Could you check a few things on this model? Use its own coordinates, in mm. A direction names the side the tool comes from. Give positions to 0.01 mm unless a question says otherwise; leave off trailing zeros. Loops run counter-clockwise (first coordinate to the right, second up) from the corner with the lowest first, then second, coordinate; pieces in that order, holes last.
1. For faces 4 (the flat face through (0, 0, 0)), 5 (the flat face through (1.926, -2.888, 4.056)), which set-ups out of +Z, -Z, +X, -X, +Y, -Y let a thin tool reach every point of the face, with its end or its side?
2. Imagine slicing it at B-B (x = -1.75). List the corners of the cut face in (y, z) for me, plus the area to 3 significant figures.
3. Thinking about a two-plate mould opening in Y: for faces 1 (the flat face through (-3.055, -1.764, 4.056)), 2 (the flat face through (0, 0, 8)), 3 (the cylindrical face through (-1.46, -6.59, 3.94)), which applies, +Y half, -Y half, draft (parallel to the pull), parting line (faces both ways), or undercut?
4. Imagine slicing it at D-D (x = -0.25). List the corners of the cut face in (y, z) for me, plus the area to 3 significant figures.
5. For P1, Ø4, axis at x = 2.5, y = 2, coming from the -Z side; P2, Ø2, axis at x = 2.5, z = 6, coming from the -Y side; P3, Ø1, axis at y = 5, z = 3.5, coming from the -X side; P4, Ø4, axis at y = 2.5, z = 5, coming from the -X side, each with a flat end and sliding along its axis, tell me the tip position at first contact or that it passes through.
6. Imagine slicing it at A-A (z = 3.5). List the corners of the cut face in (x, y) for me.
7. I need wall thicknesses on line 1 along Y through (x, z) = (3, 4.5); line 2 along Y through (x, z) = (-4.5, 4.75); line 3 along X through (y, z) = (-3.25, 1.25). Which ranges of each line are inside material? Lowest first, please.
8. Imagine slicing it at C-C (y = -4). List the corners of the cut face in (x, z) for me.
```python
from build123d import *

# Parameters (mm, degrees)
F0_R     = 6.75
F1_DEPTH = 8
F3_DEPTH = 25


with BuildPart() as f1:
    # F0 (on Top) → F1 (new body)
    with BuildSketch(Plane.XY):
        Circle(F0_R)
    extrude(amount=F1_DEPTH)

    # F2 (on face) → F3 (cut)
    with BuildSketch(Plane.XY.offset(8)):
        with BuildLine():
            ThreePointArc((0, 1.5), (0.363208, 1.455362), (0.704799, 1.324107))
            Line((0.704799, 1.324107), (2.395915, 4.950716))
            ThreePointArc((2.395915, 4.950716), (1.229036, 5.360921), (0, 5.5))
            Line((0, 5.5), (0, 1.5))
        make_face()
        with BuildLine():
            ThreePointArc((1.299038, 0.75), (1.441985, 0.413134), (1.499109, 0.051679))
            Line((1.499109, 0.051679), (5.485404, 0.400435))
            ThreePointArc((5.485404, 0.400435), (5.257212, 1.616084), (4.76314, 2.75))
            Line((4.76314, 2.75), (1.299038, 0.75))
        make_face()
        with BuildLine():
            Line((4.76314, -2.75), (1.299038, -0.75))
            ThreePointArc((1.299038, -0.75), (1.078777, -1.042229), (0.79431, -1.272427))
            Line((0.79431, -1.272427), (3.089488, -4.550281))
            ThreePointArc((3.089488, -4.550281), (4.028175, -3.744837), (4.76314, -2.75))
        make_face()
        with BuildLine():
            Line((0, -5.5), (0, -1.5))
            ThreePointArc((0, -1.5), (-0.363208, -1.455362), (-0.704799, -1.324107))
            Line((-0.704799, -1.324107), (-2.395915, -4.950716))
            ThreePointArc((-2.395915, -4.950716), (-1.229036, -5.360921), (0, -5.5))
        make_face()
        with BuildLine():
            Line((-4.76314, -2.75), (-1.299038, -0.75))
            ThreePointArc((-1.299038, -0.75), (-1.441985, -0.413134), (-1.499109, -0.051679))
            Line((-1.499109, -0.051679), (-5.485404, -0.400435))
            ThreePointArc((-5.485404, -0.400435), (-5.257212, -1.616084), (-4.76314, -2.75))
        make_face()
        with BuildLine():
            ThreePointArc((-1.299038, 0.75), (-1.078777, 1.042229), (-0.79431, 1.272427))
            Line((-0.79431, 1.272427), (-3.089488, 4.550281))
            ThreePointArc((-3.089488, 4.550281), (-4.028175, 3.744837), (-4.76314, 2.75))
            Line((-4.76314, 2.75), (-1.299038, 0.75))
        make_face()
    extrude(amount=-F3_DEPTH, mode=Mode.SUBTRACT)


solid = f1.part
```
Derived:
1. face 4: -Z, +X, -X, +Y, -Y
1. face 5: +Z, -Z
2. outline: (-6.52, 0) - (-5.21, 0) - (-5.21, 8) - (-6.52, 8) - close; (-3.57, 0) - (-1.01, 0) - (-1.01, 8) - (-3.57, 8) - close; (-0.07, 0) - (1.01, 0) - (1.01, 8) - (-0.07, 8) - close; (2.64, 0) - (6.52, 0) - (6.52, 8) - (2.64, 8) - close
2. area: 70.6 mm2
3. face 1: undercut
3. face 2: draft
3. face 3: parting line
4. outline: (-6.75, 0) - (-5.49, 0) - (-5.49, 8) - (-6.75, 8) - close; (-1.48, 0) - (6.75, 0) - (6.75, 8) - (-1.48, 8) - close
4. area: 75.8 mm2
5. P1: stops at z = 0
5. P2: stops at y = -6.58
5. P3: stops at x = -5.03
5. P4: stops at x = -6.73
6. outline: circle Ø13.5 at (0, 0); hole (-5.49, -0.4) arc R5.5 ccw to (-4.76, -2.75) - (-1.3, -0.75) arc R1.5 cw to (-1.5, -0.05) - close; hole (-4.76, 2.75) - (-1.3, 0.75) arc R1.5 cw to (-0.79, 1.27) - (-3.09, 4.55) arc R5.5 ccw to start; hole (-2.4, -4.95) arc R5.5 ccw to (0, -5.5) - (0, -1.5) arc R1.5 cw to (-0.7, -1.32) - close; hole (0, 1.5) arc R1.5 cw to (0.7, 1.32) - (2.4, 4.95) arc R5.5 ccw to (0, 5.5) - close; hole (0.79, -1.27) - (3.09, -4.55) arc R5.5 ccw to (4.76, -2.75) - (1.3, -0.75) arc R1.5 cw to start; hole (1.3, 0.75) arc R1.5 cw to (1.5, 0.05) - (5.49, 0.4) arc R5.5 ccw to (4.76, 2.75) - close
7. line 1: y = -6.05 to -4.42, -1.73 to 0.18, 1.73 to 6.05
7. line 2: y = -5.03 to -2.6, -0.31 to 2.6, 3.16 to 5.03
7. line 3: x = -5.92 to -1.6, 0 to 2.18, 4.44 to 5.92
8. outline: (-5.44, 0) - (-1.95, 0) - (-1.95, 8) - (-5.44, 8) - close; (0, 0) - (2.7, 0) - (2.7, 8) - (0, 8) - close; (3.77, 0) - (5.44, 0) - (5.44, 8) - (3.77, 8) - close
